```python
from build123d import *

# Parameters (mm, degrees)
F0_R          = 44.45
F0_R_2        = 16.51
F1_DEPTH      = 38.1
F1_DEPTH_BACK = 38.1
F8_R          = 3.175
F8_R_2        = 1.9685
F9_DEPTH      = 48.26
F10_R         = 6.35
F11_DEPTH     = 7.62
F12_R         = 3.429
F13_DEPTH     = 68.58
F14_R         = 6.35
F15_DEPTH     = 76.2


# Not quite as in the source:
# - a feature names something its author has since deleted; it is built from what else it names


with BuildPart() as f1:
    # F0 (on Top) → F1 (new body, two sides)
    with BuildSketch(Plane.XY) as f1_sk:
        with Locations((-96.7949852347, 47.625)):
            Circle(F0_R)
        with Locations((-96.7949852347, 47.625)):
            Circle(F0_R_2, mode=Mode.SUBTRACT)
        with Locations((-96.7949852347, 47.625)):
            Circle(F0_R_2)
        with BuildLine():
            ThreePointArc((-88.1051627648, 52.1100670498), (-87.4115771175, 50.37826953), (-87.0594782396, 48.5462733292))
            ThreePointArc((-87.0594782396, 48.5462733292), (-85.6757800173, 47.965243489), (-85.103715896, 46.5778145407))
            ThreePointArc((-85.103715896, 46.5778145407), (-85.8323827306, 45.0488259953), (-87.478931514, 44.6517889292))
            ThreePointArc((-87.478931514, 44.6517889292), (-88.2130581693, 42.9367840447), (-89.2595036018, 41.3923956038))
            ThreePointArc((-89.2595036018, 41.3923956038), (-88.839336444, 40.7569162622), (-88.6919210429, 40.0094919292))
            ThreePointArc((-88.6919210429, 40.0094919292), (-90.1000831422, 38.1224270954), (-92.309918185, 38.9351775301))
            ThreePointArc((-92.309918185, 38.9351775301), (-94.0417157047, 38.2415918827), (-95.8737119056, 37.8894930048))
            ThreePointArc((-95.8737119056, 37.8894930048), (-98.0529677671, 35.9450498204), (-99.7681963056, 38.3089462792))
            ThreePointArc((-99.7681963056, 38.3089462792), (-101.48320119, 39.0430729345), (-103.0275896309, 40.089518367))
            ThreePointArc((-103.0275896309, 40.089518367), (-105.9434851899, 40.2555560033), (-105.4848077047, 43.1399329502))
            ThreePointArc((-105.4848077047, 43.1399329502), (-106.178393352, 44.87173047), (-106.5304922299, 46.7037266708))
            ThreePointArc((-106.5304922299, 46.7037266708), (-108.4749354144, 48.8829825323), (-106.1110389555, 50.5982110708))
            ThreePointArc((-106.1110389555, 50.5982110708), (-105.3769123002, 52.3132159553), (-104.3304668677, 53.8576043962))
            ThreePointArc((-104.3304668677, 53.8576043962), (-104.1644292314, 56.7734999551), (-101.2800522845, 56.3148224699))
            ThreePointArc((-101.2800522845, 56.3148224699), (-99.5482547647, 57.0084081173), (-97.7162585639, 57.3605069952))
            ThreePointArc((-97.7162585639, 57.3605069952), (-95.7414309138, 59.3162590358), (-93.7792997754, 57.3477693387))
            ThreePointArc((-93.7792997754, 57.3477693387), (-93.7899471678, 57.1433056087), (-93.8217741639, 56.9410537208))
            ThreePointArc((-93.8217741639, 56.9410537208), (-92.1067692795, 56.2069270655), (-90.5623808386, 55.160481633))
            ThreePointArc((-90.5623808386, 55.160481633), (-88.4202847093, 55.5757742752), (-87.210977164, 53.7595641919))
            ThreePointArc((-87.210977164, 53.7595641919), (-87.4489020941, 52.8214265806), (-88.1051627648, 52.1100670498))
        make_face(mode=Mode.SUBTRACT)
        with BuildLine():
            ThreePointArc((-87.478931514, 44.6517889292), (-89.0293967369, 46.7886116136), (-87.0594782396, 48.5462733292))
            ThreePointArc((-87.0594782396, 48.5462733292), (-87.4115771175, 50.37826953), (-88.1051627648, 52.1100670498))
            ThreePointArc((-88.1051627648, 52.1100670498), (-90.7124690483, 52.524684387), (-90.5623808386, 55.160481633))
            ThreePointArc((-90.5623808386, 55.160481633), (-92.1067692795, 56.2069270655), (-93.8217741639, 56.9410537208))
            ThreePointArc((-93.8217741639, 56.9410537208), (-95.9585968484, 55.3905884978), (-97.7162585639, 57.3605069952))
            ThreePointArc((-97.7162585639, 57.3605069952), (-99.5482547647, 57.0084081173), (-101.2800522845, 56.3148224699))
            ThreePointArc((-101.2800522845, 56.3148224699), (-101.0424845928, 55.8008459714), (-100.9610494266, 55.2405080708))
            ThreePointArc((-100.9610494266, 55.2405080708), (-102.1821250936, 53.4194234719), (-104.3304668677, 53.8576043962))
            ThreePointArc((-104.3304668677, 53.8576043962), (-105.3769123002, 52.3132159553), (-106.1110389555, 50.5982110708))
            ThreePointArc((-106.1110389555, 50.5982110708), (-104.988766028, 49.9120186247), (-104.5492545734, 48.6721854593))
            ThreePointArc((-104.5492545734, 48.6721854593), (-105.1303256251, 47.2757495806), (-106.5304922299, 46.7037266708))
            ThreePointArc((-106.5304922299, 46.7037266708), (-106.178393352, 44.87173047), (-105.4848077047, 43.1399329502))
            ThreePointArc((-105.4848077047, 43.1399329502), (-103.4723556943, 43.221010878), (-102.4419933055, 41.4904358081))
            ThreePointArc((-102.4419933055, 41.4904358081), (-102.5942832222, 40.7312433534), (-103.0275896309, 40.089518367))
            ThreePointArc((-103.0275896309, 40.089518367), (-101.48320119, 39.0430729345), (-99.7681963056, 38.3089462792))
            ThreePointArc((-99.7681963056, 38.3089462792), (-97.6377069641, 39.8600832689), (-95.8736706941, 37.9022306613))
            ThreePointArc((-95.8736706941, 37.9022306613), (-95.873680997, 37.8958617997), (-95.8737119056, 37.8894930048))
            ThreePointArc((-95.8737119056, 37.8894930048), (-94.0417157047, 38.2415918827), (-92.309918185, 38.9351775301))
            ThreePointArc((-92.309918185, 38.9351775301), (-91.8953008477, 41.5424838136), (-89.2595036018, 41.3923956038))
            ThreePointArc((-89.2595036018, 41.3923956038), (-88.2130581693, 42.9367840447), (-87.478931514, 44.6517889292))
        make_face()
    extrude(amount=F1_DEPTH)
    extrude(f1_sk.sketch, amount=-F1_DEPTH_BACK)

    # F2 (on Top) → F3 (revolve, cut)
    with BuildSketch(Plane.XY):
        with BuildLine():
            Line((-32.5839432458, 95.377), (-32.5839432458, 47.625))
            Line((-32.5839432458, 47.625), (-32.5839432458, -0.127))
            Line((-32.5839432458, -0.127), (-32.5839432458, -9.525))
            ThreePointArc((-32.5839432458, -9.525), (15.1680567542, 47.625), (-32.5839432458, 104.775))
            Line((-32.5839432458, 104.775), (-32.5839432458, 95.377))
        make_face()
    revolve(axis=Axis((-32.5839432458, 19.05, 0), (0, -1, 0)), mode=Mode.SUBTRACT)

    # F4 (on Top) → F5 (revolve, cut)
    with BuildSketch(Plane.XY):
        with BuildLine():
            Line((-88.4089947582, -28.0660327723), (-131.1163690465, -6.7040645718))
            Line((-131.1163690465, -6.7040645718), (-173.8237433348, 14.6579036287))
            ThreePointArc((-173.8237433348, 14.6579036287), (-152.478337247, -49.4114388601), (-88.4089947582, -28.0660327723))
        make_face()
    revolve(axis=Axis((-152.4700561907, 3.9769195285, 0), (-0.894357813, 0.4473523245, 0)), mode=Mode.SUBTRACT)

    # F6 (on Top) → F7 (revolve, cut)
    with BuildSketch(Plane.XY):
        with BuildLine():
            ThreePointArc((-83.0436281881, 123.89609931), (-146.068020162, 148.1537377837), (-170.3256586357, 85.1293458098))
            Line((-170.3256586357, 85.1293458098), (-126.6846434119, 104.5127225599))
            Line((-126.6846434119, 104.5127225599), (-83.0436281881, 123.89609931))
        make_face()
    revolve(axis=Axis((-148.5051510238, 94.8210341849, 0), (0.9139096839, 0.4059175898, 0)), mode=Mode.SUBTRACT)

    # F8 (on face) → F9 (cut)
    with BuildSketch(Plane.XY.offset(38.1)):
        with Locations((-102.9295494266, 55.2405080708)):
            Circle(F8_R)
        with Locations((-102.9295494266, 55.2405080708)):
            Circle(F8_R_2, mode=Mode.SUBTRACT)
        with Locations((-95.7477997754, 57.3477693387)):
            Circle(F8_R)
        with Locations((-95.7477997754, 57.3477693387)):
            Circle(F8_R_2, mode=Mode.SUBTRACT)
        with Locations((-89.179477164, 53.7595641919)):
            Circle(F8_R)
        with Locations((-89.179477164, 53.7595641919)):
            Circle(F8_R_2, mode=Mode.SUBTRACT)
        with Locations((-87.072215896, 46.5778145407)):
            Circle(F8_R)
        with Locations((-87.072215896, 46.5778145407)):
            Circle(F8_R_2, mode=Mode.SUBTRACT)
        with Locations((-90.6604210429, 40.0094919292)):
            Circle(F8_R)
        with Locations((-90.6604210429, 40.0094919292)):
            Circle(F8_R_2, mode=Mode.SUBTRACT)
        with Locations((-97.8421706941, 37.9022306613)):
            Circle(F8_R)
        with BuildLine():
            ThreePointArc((-95.8736706941, 37.9022306613), (-95.873680997, 37.8958617997), (-95.8737119056, 37.8894930048))
            ThreePointArc((-95.8737119056, 37.8894930048), (-99.8106603912, 37.9085995228), (-95.8736706941, 37.9022306613))
        make_face(mode=Mode.SUBTRACT)
        with Locations((-104.4104933055, 41.4904358081)):
            Circle(F8_R)
        with Locations((-104.4104933055, 41.4904358081)):
            Circle(F8_R_2, mode=Mode.SUBTRACT)
        with Locations((-106.5177545734, 48.6721854593)):
            Circle(F8_R)
        with Locations((-106.5177545734, 48.6721854593)):
            Circle(F8_R_2, mode=Mode.SUBTRACT)
    extrude(amount=-F9_DEPTH, mode=Mode.SUBTRACT)

    # F10 (on face) → F11 (cut)
    with BuildSketch(Plane.XY.offset(38.1)):
        with Locations((-96.7949852347, 47.625)):
            Circle(F10_R)
    extrude(amount=-F11_DEPTH, mode=Mode.SUBTRACT)

    # F12 (on face) → F13 (cut, through all)
    with BuildSketch(Plane.XY.offset(30.48)):
        with Locations((-96.7949852347, 47.625)):
            Circle(F12_R)
    extrude(amount=-F13_DEPTH, mode=Mode.SUBTRACT)

    # F14 (on face) → F15 (cut, through all)
    with BuildSketch(Plane.XY.offset(38.1)):
        with Locations((-127.8890646346, 48.8640254414)):
            Circle(F14_R)
        with BuildLine():
            ThreePointArc((-76.7834769385, 79.3022345884), (-85.5434026681, 77.325191035), (-83.5663591148, 68.5652653054))
            Line((-83.5663591148, 68.5652653054), (-76.7834769385, 79.3022345884))
        make_face()
        with BuildLine():
            Line((-76.7834769385, 79.3022345884), (-83.5663591148, 68.5652653054))
            ThreePointArc((-83.5663591148, 68.5652653054), (-77.1100486093, 68.3723584434), (-73.8249180267, 73.9337499469))
            ThreePointArc((-73.8249180267, 73.9337499469), (-74.6135265232, 76.9986193642), (-76.7834769385, 79.3022345884))
        make_face()
        with Locations((-82.3209730429, 20.0772246117)):
            Circle(F14_R)
    extrude(amount=-F15_DEPTH, mode=Mode.SUBTRACT)


solid = f1.part
```
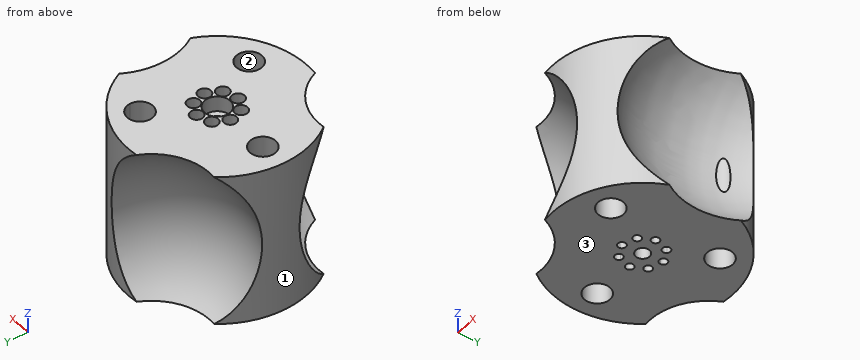
Here's how the part is built. I have some questions about the finished solid (model axes, mm). Face numbers are marked on the shaded views. Coordinates: 2 decimals unless noted, no trailing zeros. Write each loop counter-clockwise with the first axis right and the second up, starting at its lowest first coordinate (ties: lowest second). Pieces come first, ordered by that corner, then holes. Notation, with made-up numbers: (-19.5, 14) -> (39.5, 14) arc R15 cw to (39.5, 41) -> close; hole circle Ø3 at (-12, 47.25). An arc over 180 degrees is marked (long way). Use a Markdown table: item, result. Add a question column.
(1) I'm going to push flat-ended pins straight in: P1, Ø3.5, axis at x = -102.93, y = 55.24, coming from the +Z side; P2, Ø3, axis at x = -97, y = 38, coming from the +Z side; P3, Ø8, axis at y = 50, z = 15.5, coming from the -X side (3 decimals); P4, Ø10, axis at x = -68, z = -22, coming from the +Y side. Where does each tip first touch, or does it pass through?
(2) If we section it at B-B, the plane y = 72: State how many separate pieces and enclosed holes the cut face has, and give its area (3 significant figures).
(3) Please list where these lines run through material, in increasing order: line 1 (X direction, y = 57, z = 20.5); line 2 (X direction, y = 54, z = -31); line 3 (Y direction, x = -96.5, z = -2.5).
(4) We'd pull the mould along X, two halves only. Please class the marked faces 1, 2 and 3: +X half, -X half, draft (parallel to the pull), parting line (faces both ways), or undercut.
(5) If we section it at A-A, the plane x = -126: Write out the boundary of the cut face in (y, z), and give its area (3 significant figures).
Outcome:
| question | item | result |
|---|---|---|
| 1 | P1 | passes through |
| 1 | P2 | stops at z = -10.16 |
| 1 | P3 | stops at x = -141.245 |
| 1 | P4 | stops at y = 85.17 |
| 2 | separate pieces | 3 |
| 2 | enclosed holes | 0 |
| 2 | area | 1,630 mm^2 |
| 3 | line 1 | x = -140.25 to -105.57, -100.29 to -98.9, -92.59 to -74.87 |
| 3 | line 2 | x = -140.79 to -131.62, -124.15 to -104.46, -101.4 to -91.13, -87.23 to -68.44 |
| 3 | line 3 | y = 26.09 to 35.02, 40.78 to 44.21, 51.04 to 54.26, 60.43 to 67.6 |
| 4 | face 1 | -X half |
| 4 | face 2 | undercut |
| 4 | face 3 | draft |
| 5 | outline | (21.62, -38.1) -> (42.8, -38.1) -> (42.8, 38.1) -> (21.62, 38.1) arc R47.48 cw to start; (54.93, -38.1) -> (75.73, -38.1) arc R47.75 cw to (75.73, 38.1) -> (54.93, 38.1) -> close |
| 5 | area | 1,170 mm^2 |
